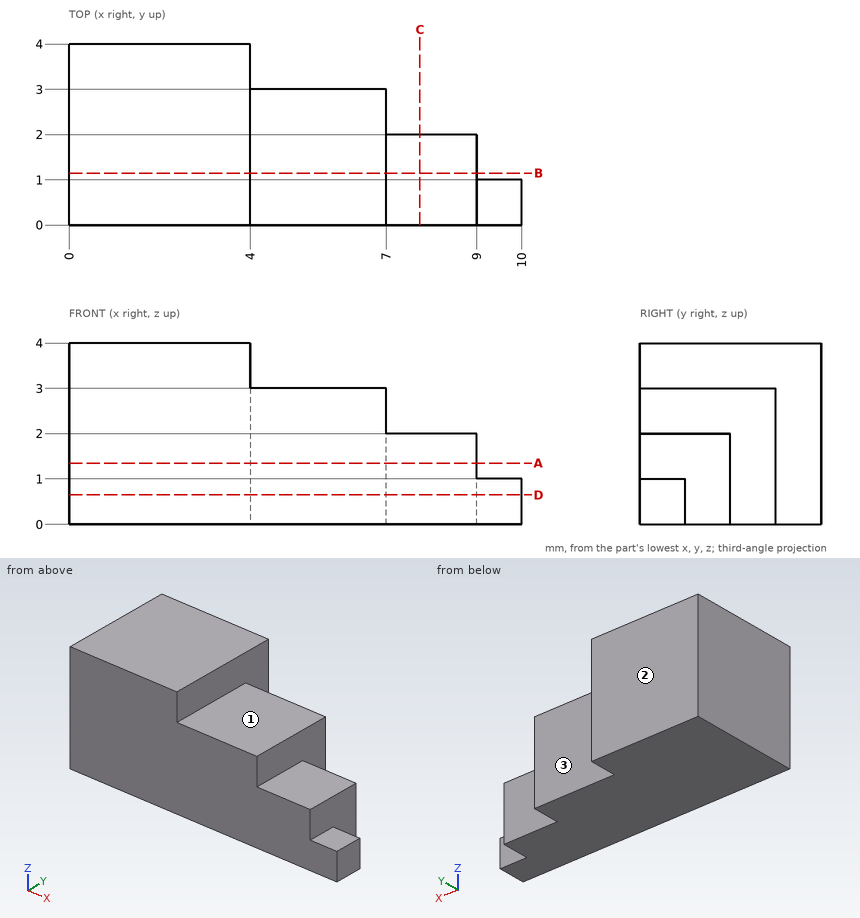
Here's the drawing with two shaded views (mm, measured from the low corner). I have some questions. A direction names the side the tool comes from. Coordinates: 2 decimals unless noted, no trailing zeros. Write each loop counter-clockwise with the first axis right and the second up, starting at its lowest first coordinate (ties: lowest second). Pieces come first, ordered by that corner, then holes. Notation, with made-up numbers: (51.5, 38.5) -> (65.5, 38.5) arc R31 cw to (65.5, 71.5) -> close; hole circle Ø11 at (53.25, 42). An arc over 180 degrees is marked (long way). Use a Markdown table: item, result. Add a question column.
(1) For the marked faces 1, 2 and 3, which set-ups out of +Z, -Z, +X, -X, +Y, -Y let a thin tool reach every point of the face, with its end or its side?
(2) I'm going to push flat-ended pins straight in: P1, Ø0.5, axis at x = 9.5, z = 0.5, coming from the +Y side; P2, Ø1.5, axis at y = 3, z = 3, coming from the +X side; P3, Ø0.8, axis at x = 9.5, y = 0.5, coming from the +Z side; P4, Ø2, axis at y = 1, z = 1.5, coming from the +X side. Where does each tip first touch, or does it pass through?
(3) If we section it at D-D, the plane z = 0.65: Write out the boundary of the cut face in (x, y), and give its area (3 significant figures).
(4) If we section it at A-A, the plane z = 1.35: Write out the boundary of the cut face in (x, y).
(5) Please list where these lines run through material, in increasing order: line 1 (X direction, y = 2.8, z = 1.9); line 2 (Y direction, x = 8.5, z = 1.65); line 3 (Y direction, x = 6.25, z = 2).
(6) If we section it at C-C, the plane x = 7.75: Write out the boundary of the cut face in (y, z), and give its area (3 significant figures).
Outcome:
| question | item | result |
|---|---|---|
| 1 | face 1 | +Z, +X, +Y, -Y |
| 1 | face 2 | +Z, -Z, +X, -X, +Y |
| 1 | face 3 | +Z, -Z, +X, +Y |
| 2 | P1 | stops at y = 1 |
| 2 | P2 | stops at x = 7 |
| 2 | P3 | stops at z = 1 |
| 2 | P4 | stops at x = 10 |
| 3 | outline | (0, 0) -> (10, 0) -> (10, 1) -> (9, 1) -> (9, 2) -> (7, 2) -> (7, 3) -> (4, 3) -> (4, 4) -> (0, 4) -> close |
| 3 | area | 30.0 mm^2 |
| 4 | outline | (0, 0) -> (9, 0) -> (9, 2) -> (7, 2) -> (7, 3) -> (4, 3) -> (4, 4) -> (0, 4) -> close |
| 5 | line 1 | x = 0 to 7 |
| 5 | line 2 | y = 0 to 2 |
| 5 | line 3 | y = 0 to 3 |
| 6 | outline | (0, 0) -> (2, 0) -> (2, 2) -> (0, 2) -> close |
| 6 | area | 4.00 mm^2 |
